Part print with two shaded views. Sizes in mm from the minimum x, y, z corner. A direction names the side the tool comes from. Round coordinates to 2 decimals unless told otherwise and drop trailing zeros. Order: outer loops, then holes, each group sorted by start corner. A loop starts at its lowest first (then second) coordinate and runs counter-clockwise, first axis right, second up. Notation, with made-up numbers: (76, -30) -> (116, -30) arc R25 ccw to (116, -18) -> close; hole circle Ø6 at (58, 37.25). An arc over 180 degrees is marked (long way). Put each result on its own line as item: value. Start each with the question number.
Q1. Cut at A-A, the plane x = 15. List the corners of the cut face in (y, z).
Q2. Cut at B-B, the plane z = 49.5. List the corners of the cut face in (x, y).
Q3. Cut at D-D, the plane y = 18. List the corners of the cut face in (x, z), and give its area (3 significant figures).
Q4. Cut at C-C, the plane z = 40. List the corners of the cut face in (x, y).
Q5. 3-axis set-ups, long thin cutter, end or side, ignore diameter. For the marked faces 1 and 2: which of +Z, -Z, +X, -X, +Y, -Y reach the whole face in a straight line?
Q6. Flat gauge pin, fed straight in: P1, Ø12, axis at x = 70, y = 20.5, coming from the +Z side. Where does the tip first touch, or does it go through?
Q7. Probe L1, parallel to Z at x = 15, y = 8.25; L2, parallel to X at y = 8.5, z = 29.5; L3, parallel to Z at x = 53.5, y = 13. List the from-to ranges inside material, lowest first.
Q8. Pull direction X, two halves, no side cores. Call the marked faces 3, 4 and 5: released by +X, released by -X, zero draft, split by the parting line, or undercut.
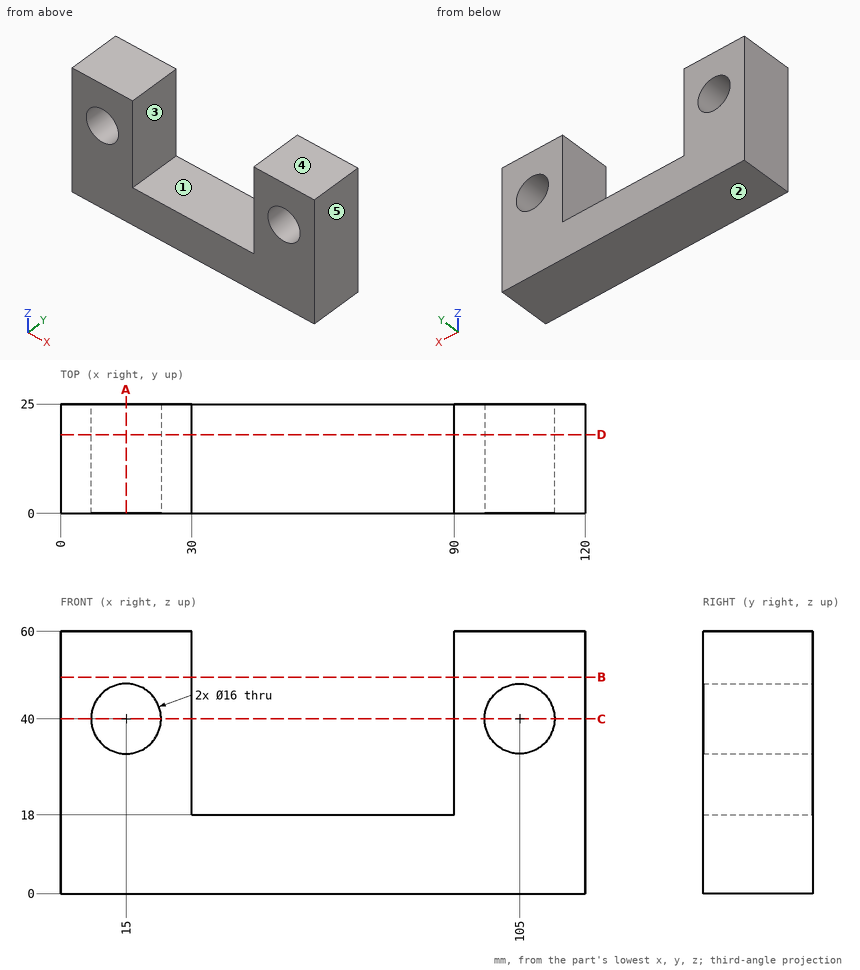
Ans:
1. outline: (0, 0) -> (25, 0) -> (25, 32) -> (0, 32) -> close; (0, 48) -> (25, 48) -> (25, 60) -> (0, 60) -> close
2. outline: (0, 0) -> (30, 0) -> (30, 25) -> (0, 25) -> close; (90, 0) -> (120, 0) -> (120, 25) -> (90, 25) -> close
3. outline: (0, 0) -> (120, 0) -> (120, 60) -> (90, 60) -> (90, 18) -> (30, 18) -> (30, 60) -> (0, 60) -> close; hole circle Ø16 at (15, 40); hole circle Ø16 at (105, 40)
3. area: 4,280 mm^2
4. outline: (0, 0) -> (7, 0) -> (7, 25) -> (0, 25) -> close; (23, 0) -> (30, 0) -> (30, 25) -> (23, 25) -> close; (90, 0) -> (97, 0) -> (97, 25) -> (90, 25) -> close; (113, 0) -> (120, 0) -> (120, 25) -> (113, 25) -> close
5. face 1: +Z, +Y, -Y
5. face 2: -Z, +X, -X, +Y, -Y
6. P1: stops at z = 18
7. L1: z = 0 to 32, 48 to 60
7. L2: x = 0 to 30, 90 to 120
7. L3: z = 0 to 18
8. face 3: undercut
8. face 4: zero draft
8. face 5: released by +X
